```python
from build123d import *

# Parameters (mm, degrees)
CUT_EXTRUDE1_REACH = 18
SKETCH3_R          = 3


with BuildPart() as part:
    # Sketch1 → Revolve1 (revolve)
    with BuildSketch(Plane(origin=(0, 0, 0), x_dir=(1, 0, 0), z_dir=(0, 1, 0))):
        Polygon((-54.771838843, 0), (-54.771838843, 6), (-45.771838843, 6), (-45.771838843, 3), (-39.771838843, 3), (-39.771838843, 6), (-32.771838843, 6), (-32.771838843, 8), (49.228161157, 8), (49.228161157, 6), (59.228161157, 6), (59.228161157, 8), (83.228161157, 8), (83.228161157, 0), align=None)
    revolve(axis=Axis((-54.771838843, 0, 0), (1, 0, 0)))

    # Sketch3 → Cut-Extrude1 (cut, up to next)
    with BuildSketch(Plane(origin=(0, 8, 0), x_dir=(1, 0, 0), z_dir=(0, 1, 0)), mode=Mode.PRIVATE) as cut_extrude1_sk1:
        with Locations((71.228161157, 0)):
            Circle(SKETCH3_R)
    cut_extrude1_tool1 = extrude(cut_extrude1_sk1.sketch, amount=-CUT_EXTRUDE1_REACH, mode=Mode.PRIVATE) & part.part
    add(cut_extrude1_tool1.solids().sort_by_distance((71.228161, 8, 0))[0], mode=Mode.SUBTRACT)


solid = part.part
```
Input: part model. Units: mm. Frame: model coordinates. A direction names the side the tool comes from. Coordinates: 2 decimals unless noted, no trailing zeros. Loops run counter-clockwise (first coordinate to the right, second up) from the corner with the lowest first, then second, coordinate; pieces in that order, holes last. Notation, with made-up numbers: M 59.5,17 L 81.5,17 A8 cw 81.5,23 Z; hole C -35.5,12.25 d2. An arc over 180 degrees is marked long. Use a Markdown table: item, result. Add a question column.
1) Pin query (flat end, axial travel): P1, Ø4, axis at x = 65, y = -3, coming from the -Z side; P2, Ø3.5, axis at x = 71.23, z = 0, coming from the -Y side; P3, Ø5, axis at x = -37, y = 6, coming from the -Z side; P4, Ø6, axis at x = 25, z = 5, coming from the -Y side. Return the tip coordinate at first contact, or that it passes through.
2) Set-up query: faces 4 (the flat face through (-32.772, 6, -2)), 5 (the cylindrical face through (8.8, -7.81, 1.73)), 6 (the flat face through (49.228, 6, 2)). Return all of +Z, -Z, +X, -X, +Y, -Y with unobstructed straight access to the full face (end or side cutting, diameter ignored); none if empty.
3) Section A-A, the plane z = 0. Return the cut outline in (x, y), plus the area to 3 significant figures.
4) Section B-B, the plane y = 0. Return the cut outline in (x, z).
5) Draft query along Z for faces 1 (the cylindrical face through (68.85, 0.11, 1.83)), 2 (the cylindrical face through (71.4, -7.1, -3.69)), 3 (the flat face through (-39.772, -1, -3)). Return one class per face: +Z half, -Z half, draft (parallel to the pull), parting line (faces both ways), or undercut.
6) Line query: L1, parallel to X at y = -3.25, z = 0; L2, parallel to X at y = -2.5, z = -3.25; L3, parallel to X at y = 0, z = 0. Output: solid intervals per line, ascending. Write a range as from..to.
7) Section C-C, the plane x = -25.5. Return the cut outline in (y, z).
Answer below:
| question | item | result |
|---|---|---|
| 1 | P1 | z = -7.94 |
| 1 | P2 | through |
| 1 | P3 | z = -4.87 |
| 1 | P4 | y = -7.75 |
| 2 | face 4 | -X |
| 2 | face 5 | +X, -X |
| 2 | face 6 | none |
| 3 | outline | M -54.77,-6 L -45.77,-6 L -45.77,-3 L -39.77,-3 L -39.77,-6 L -32.77,-6 L -32.77,-8 L 49.23,-8 L 49.23,-6 L 59.23,-6 L 59.23,-8 L 68.23,-8 L 68.23,8 L 59.23,8 L 59.23,6 L 49.23,6 L 49.23,8 L -32.77,8 L -32.77,6 L -39.77,6 L -39.77,3 L -45.77,3 L -45.77,6 L -54.77,6 Z; M 74.23,-8 L 83.23,-8 L 83.23,8 L 74.23,8 Z |
| 3 | area | 1,950 mm2 |
| 4 | outline | M -54.77,-6 L -45.77,-6 L -45.77,-3 L -39.77,-3 L -39.77,-6 L -32.77,-6 L -32.77,-8 L 49.23,-8 L 49.23,-6 L 59.23,-6 L 59.23,-8 L 83.23,-8 L 83.23,8 L 59.23,8 L 59.23,6 L 49.23,6 L 49.23,8 L -32.77,8 L -32.77,6 L -39.77,6 L -39.77,3 L -45.77,3 L -45.77,6 L -54.77,6 Z; hole C 71.23,0 d6 |
| 5 | face 1 | undercut |
| 5 | face 2 | parting line |
| 5 | face 3 | draft |
| 6 | L1 | -54.77..-45.77, -39.77..68.23, 74.23..83.23 |
| 6 | L2 | -54.77..-45.77, -39.77..83.23 |
| 6 | L3 | -54.77..68.23, 74.23..83.23 |
| 7 | outline | C 0,0 d16 |
